Geometry check sheet. Reference: drawing and pictorial views, mm from the part's lowest x, y, z. A direction names the side the tool comes from. Give positions to 0.01 mm unless a question says otherwise; leave off trailing zeros. Write each loop counter-clockwise with the first axis right and the second up, starting at its lowest first coordinate (ties: lowest second). Pieces come first, ordered by that corner, then holes. Notation, with made-up numbers: (3, 20) -> (62, 20) arc R27 ccw to (62, 55) -> close; hole circle Ø11 at (-4, 67). An arc over 180 degrees is marked (long way). Return JSON: item names as keys, results as strings.
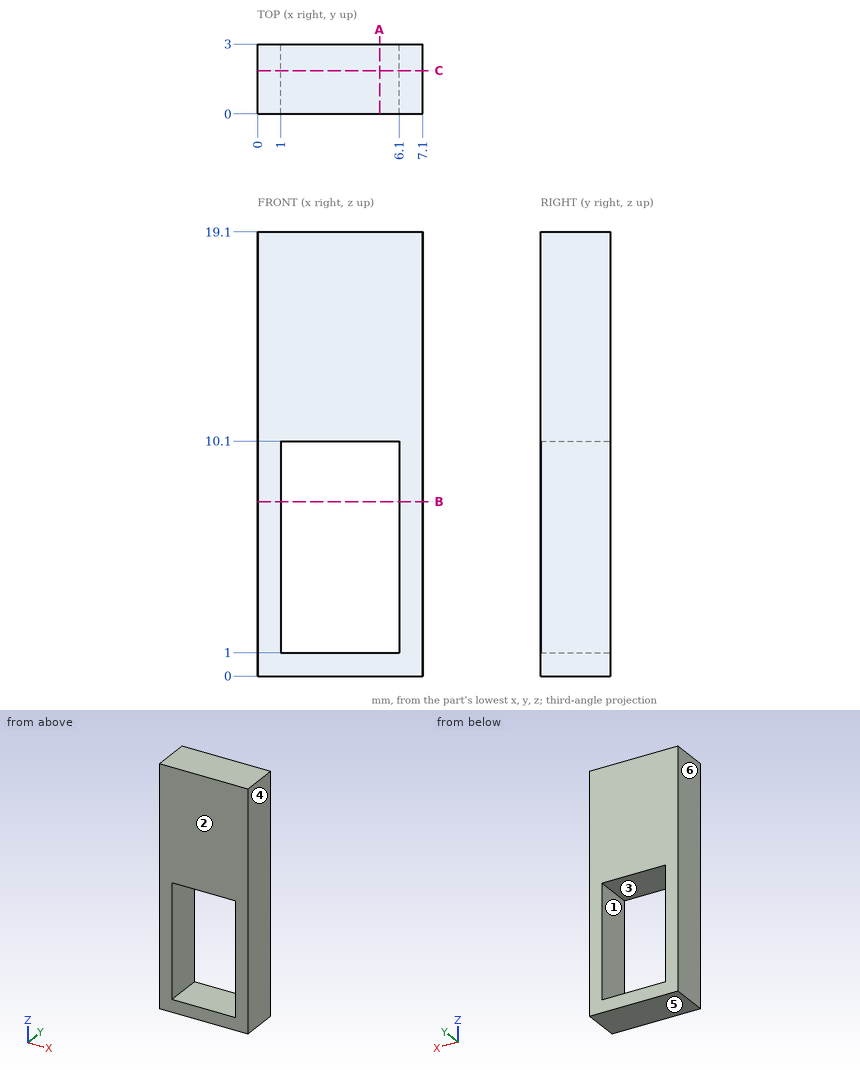
(1) Cross-section at C-C on y = 1.85. Enter the section's corners in (x, z).
Reply:
{"outline": "(0, 0) -> (7.1, 0) -> (7.1, 19.1) -> (0, 19.1) -> close; hole (1, 1) -> (6.1, 1) -> (6.1, 10.1) -> (1, 10.1) -> close"}
(2) Thickness scan on L1, parallel to Z at x = 2.5, y = 1.3; L2, parallel to X at y = 0.85, z = 9.75. Record the ranges inside material, lowest first.
Reply:
{"L1": "0 to 1, 10.1 to 19.1", "L2": "0 to 1, 6.1 to 7.1"}
(3) Release check for a two-part mould opening along X. For the marked faces 3, 4, 5 and 6 record: pulls with the +X half, pulls with the -X half, needs draft (parallel to the pull), parting line crosses it, or undercut.
Reply:
{"face 3": "undercut", "face 4": "pulls with the +X half", "face 5": "needs draft", "face 6": "pulls with the -X half"}
(4) Cross-section at B-B on z = 7.5. Enter the section's corners in (x, y), then the cut area to 3 significant figures.
Reply:
{"outline": "(0, 0) -> (1, 0) -> (1, 3) -> (0, 3) -> close; (6.1, 0) -> (7.1, 0) -> (7.1, 3) -> (6.1, 3) -> close", "area": "6.00 mm^2"}
(5) Set-up check for the marked faces 1 and 2: record each of +Z, -Z, +X, -X, +Y, -Y from which the full face is reachable in a straight line by a thin tool's end or side.
Reply:
{"face 1": "+Y, -Y", "face 2": "+Z, -Z, +X, -X, -Y"}
(6) Cross-section at A-A on x = 5.25. Enter the section's corners in (y, z).
Reply:
{"outline": "(0, 0) -> (3, 0) -> (3, 1) -> (0, 1) -> close; (0, 10.1) -> (3, 10.1) -> (3, 19.1) -> (0, 19.1) -> close"}
